Geometry check sheet. Reference: the model listing, model coordinates, mm. A direction names the side the tool comes from. Round coordinates to 2 decimals unless told otherwise and drop trailing zeros. Write each loop counter-clockwise with the first axis right and the second up, starting at its lowest first coordinate (ties: lowest second). Pieces come first, ordered by that corner, then holes. Notation, with made-up numbers: (79.5, 43.25) -> (90.5, 43.25) arc R30 cw to (90.5, 74.25) -> close; hole circle Ø2 at (-36, -10). An arc over 180 degrees is marked (long way). Use a Markdown table: item, result.
Autodesk Inventor part; units mm, degrees
ref_plane "YZ Plane" through (0, 0, 0) normal (1, 0, 0) x (0, 1, 0)
ref_plane "XZ Plane" through (0, 0, 0) normal (0, 1, 0) x (-1, 0, 0)
ref_plane "XY Plane" through (0, 0, 0) normal (0, 0, 1) x (1, 0, 0)
sketch "Эскиз1" plane through (0, 0, 0) normal (0, 0, 1) x (1, 0, 0)
  line L0 (-45, 34) -> (45, 34)
  line L1 (45, 34) -> (45, -34)
  line L2 (45, -34) -> (-45, -34)
  line L3 (-45, -34) -> (-45, 34)
  point P0 (0, 0)
  point P1 (-45, 0)
  point P2 (0, 34)
  dimension "d0" = 90
  dimension "d1" = 68
extrude "Выдавливание1" add sketch "Эскиз1" against normal blind 40
sketch "Эскиз2" plane through (0, 0, 0) normal (0, 0, 1) x (1, 0, 0)
  line L0 (-45, -34) -> (-45, 34)
  line L1 (-45, 20) -> (-27.5, 20)
  line L2 (-27.5, 20) -> (-13.5, 34)
  line L3 (-13.5, 34) -> (13.5, 34)
  line L4 (-45, 34) -> (45, 34)
  line L5 (13.5, 34) -> (27.5, 20)
  line L6 (27.5, 20) -> (45, 20)
  line L7 (45, 34) -> (45, -34)
  line L8 (45, -34) -> (-45, -34)
  point P0 (0, 0)
  dimension "d4" = 27
  dimension "d5" = 55
  dimension "d6" = 17.5
  dimension "d7" = 14
  dimension "d8" = 54
  dimension "d9" = 135
extrude "Выдавливание2" cut sketch "Эскиз2" against normal blind 40 contours L0 L4 L2 L1 | L6 L5 L4 L7
sketch "Эскиз3" plane through (0, 0, 0) normal (0, 0, 1) x (1, 0, 0)
  line L0 (-45, 20) -> (-27.5, 20)
  line L1 (-43.5, 20) -> (-43.5, -24.5)
  line L2 (-43.5, -24.5) -> (-45, -26)
  line L3 (-45, -34) -> (-45, 20)
  line L4 (45, -34) -> (-45, -34)
  point P0 (0, 0)
  dimension "d12" = 1.5
  dimension "d13" = 1.5
  dimension "d14" = 8
extrude "Выдавливание3" cut sketch "Эскиз3" against normal blind 40
sketch "Эскиз5" plane through (0, 0, 0) normal (0, 0, 1) x (1, 0, 0)
  line L0 (27.5, 20) -> (45, 20)
  line L1 (43.5, 20) -> (43.5, -24.5)
  line L2 (43.5, -24.5) -> (45, -26)
  line L3 (45, 20) -> (45, -34)
  point P0 (0, 0)
  point P1 (-43.5, -24.5)
  point P2 (-45, -26)
  dimension "d21" = 1.5
extrude "Выдавливание4" cut sketch "Эскиз5" against normal blind 40
sketch "Эскиз6" plane through (0, 0, 0) normal (0, 0, 1) x (1, 0, 0)
  circle A0 centre (0, 0) radius 26
  line L0 (25.9567, 1.5) -> (43.5, 1.5)
  line L1 (43.5, 20) -> (43.5, -24.5)
  line L2 (25.9567, -1.5) -> (43.5, -1.5)
  line L3 (45, -34) -> (-45, -34)
  point P0 (0, -26)
  dimension "d24" = 52
  dimension "d25" = 8
  dimension "d26" = 3
  dimension "d27" = 1.5
extrude "Выдавливание5" cut sketch "Эскиз6" against normal blind 40
sketch "Эскиз7" plane through (-45, -34, 0) normal (0, -1, 0) x (1, 0, 0)
  line L0 (90, 0) -> (0, 0)
  line L1 (0, 0) -> (0, -40)
  point P0 (45, 0)
  point P1 (80, -30)
  point P2 (80, -10)
  point P3 (10, -10)
  point P4 (10, -30)
  dimension "d30" = 20
  dimension "d31" = 70
  dimension "d32" = 10
  dimension "d33" = 10
hole "Отверстие1" at (35, -34, -30) at (35, -34, -10) at (-35, -34, -10) at (-35, -34, -30) direction (0, 1, 0) diameter 6.5 end through all
chamfer "Фаска1" distance 0.5 angle 45 10 edges at (35, 20, -26.75) (35, 20, -6.75) (-35, 20, -26.75) (-35, 20, -6.75) (-26, 0, -40) (-26, 0, 0) (35, -34, -26.75) (-35, -34, -26.75) (35, -34, -6.75) (-35, -34, -6.75)
sketch "Эскиз8" plane through (0, 0, 0) normal (0, 0, 1) x (1, 0, 0)
  line L0 (45, -34) -> (-45, -34)
  line L1 (-27.5, -34) -> (-26.5, -33)
  line L2 (-26.5, -33) -> (-14.5, -33)
  line L3 (-14.5, -33) -> (-13.5, -34)
  line L4 (13.5, -34) -> (14.5, -33)
  line L5 (14.5, -33) -> (26.5, -33)
  line L6 (26.5, -33) -> (27.5, -34)
  point P0 (0, 0)
  point P1 (-27.5, 20)
  point P2 (-13.5, 34)
  point P3 (13.5, 34)
  point P4 (27.5, 20)
  dimension "d44" = 1
  dimension "d45" = 45
  dimension "d46" = 45
  dimension "d47" = 45
extrude "Выдавливание6" cut sketch "Эскиз8" against normal blind 40
properties part number "SMK52"
(1) Section check C-C on y = 0. Record the cut outline in (x, z).
A:
| item | result |
|---|---|
| outline | (-43.5, -40) -> (-26.5, -40) -> (-26, -39.5) -> (-26, -0.5) -> (-26.5, 0) -> (-43.5, 0) -> close; hole circle Ø6.5 at (-35, -30); hole circle Ø6.5 at (-35, -10) |
(2) Access from +Z, -Z, +X, -X, +Y, -Y to the whole of each face (thin tool, end or side, straight path). Record for faces 1 (the face through (35, -1.5, -20)), 2 (the face through (36, -34, -20)), 3 (the face through (43.5, -13, -20)).
A:
| item | result |
|---|---|
| face 1 | +Z, -Z, +X |
| face 2 | +Z, -Z, +X, -X, -Y |
| face 3 | +Z, -Z, +X, +Y |
(3) Release check for a two-part mould opening along Z. For faces 4 (the face through (-26.118, 1.129, -0.358)), 5 (the face through (37.883, -17.276, -31.5)), 6 (the face through (38.173, -17.276, -9.295)), 7 (the face through (-45, -30, -20)) record: +Z half, -Z half, draft (parallel to the pull), parting line (faces both ways), or undercut.
A:
| item | result |
|---|---|
| face 4 | +Z half |
| face 5 | undercut |
| face 6 | undercut |
| face 7 | draft |
(4) Thickness scan on line 1 (Z direction, x = 35, y = -23); line 2 (X direction, y = 15, z = -10); line 3 (X direction, y = -8, z = -32). Record the ranges inside material, lowest first.
A:
| item | result |
|---|---|
| line 1 | z = -40 to -33.25, -26.75 to -13.25, -6.75 to 0 |
| line 2 | x = -43.5 to -38.25, -31.75 to -21.24, 21.24 to 31.75, 38.25 to 43.5 |
| line 3 | x = -43.5 to -37.56, -32.44 to -24.74, 24.74 to 32.44, 37.56 to 43.5 |
(5) Gauge pin test, flat ends, axial feed: pin 1 Ø4 at (x, z) = (35, -30) entering from -Y; pin 2 Ø8.5 at (x, z) = (-35, -10) entering from +Y; pin 3 Ø5.5 at (y, z) = (13, -27.5) entering from +X; pin 4 Ø3.5 at (x, z) = (-20.5, -25.5) entering from -Y. Record the tip position at first contact, or that the pin passes through.
A:
| item | result |
|---|---|
| pin 1 | passes through |
| pin 2 | stops at y = 20 |
| pin 3 | stops at x = 43.5 |
| pin 4 | stops at y = -33 |
(6) Section check A-A on x = 35. State how many separate pieces and enclosed holes the cut face has, plus the area to 3 significant figures.
A:
| item | result |
|---|---|
| separate pieces | 6 |
| enclosed holes | 0 |
| area | 1,380 mm2 |
(7) Section check B-B on x = -35. Record the cut outline in (y, z).
A:
| item | result |
|---|---|
| outline | (-34, -40) -> (20, -40) -> (20, -33.75) -> (19.5, -33.25) -> (-33.5, -33.25) -> (-34, -33.75) -> close; (-34, -26.25) -> (-33.5, -26.75) -> (19.5, -26.75) -> (20, -26.25) -> (20, -13.75) -> (19.5, -13.25) -> (-33.5, -13.25) -> (-34, -13.75) -> close; (-34, -6.25) -> (-33.5, -6.75) -> (19.5, -6.75) -> (20, -6.25) -> (20, 0) -> (-34, 0) -> close |
(8) Section check D-D on z = -18. Record the cut outline in (x, y).
A:
| item | result |
|---|---|
| outline | (-45, -34) -> (-27.5, -34) -> (-26.5, -33) -> (-14.5, -33) -> (-13.5, -34) -> (13.5, -34) -> (14.5, -33) -> (26.5, -33) -> (27.5, -34) -> (45, -34) -> (45, -26) -> (43.5, -24.5) -> (43.5, -1.5) -> (25.96, -1.5) arc R26 cw (long way) to (25.96, 1.5) -> (43.5, 1.5) -> (43.5, 20) -> (27.5, 20) -> (13.5, 34) -> (-13.5, 34) -> (-27.5, 20) -> (-43.5, 20) -> (-43.5, -24.5) -> (-45, -26) -> close |
